CAD build for the part. Positions are in the model's coordinates, mm. Face numbers are marked on the shaded views. Round coordinates to 2 decimals unless told otherwise and drop trailing zeros. Order: outer loops, then holes, each group sorted by start corner. A loop starts at its lowest first (then second) coordinate and runs counter-clockwise, first axis right, second up. Notation, with made-up numbers: (21, -4.75) -> (67, -4.75) arc R22 ccw to (67, 32.25) -> close; hole circle Ø3 at (-39.5, 56). An arc over 180 degrees is marked (long way). Answer as CSV lines item,"result". Start each with the question number.
from build123d import *

# Parameters (mm, degrees)
SKETCH004_W          = 7
SKETCH004_H          = 3
SKETCH005_W          = 7
SKETCH005_H          = 3
POCKET_DEPTH         = 12.001
POCKET001_DEPTH      = 12.001
SKETCH009_W          = 7
SKETCH009_H          = 3
SKETCH010_W          = 7
SKETCH010_H          = 3
POCKET002_DEPTH      = 6.001
POCKET002_DEPTH_BACK = -6.001


with BuildPart() as part:
    # AdditivePipe: sweep along a path in Sketch002
    with BuildLine(Plane.XY) as additivepipe_path:
        ThreePointArc((0, 0), (-10.865453, 68.601773), (-42.398227, 130.488326))
    # Sketch → AdditivePipe (sweep)
    with BuildSketch(Plane.XZ):
        Polygon((-20, 6), (-20, -6), (-16, -6), (-16, -3), (-9, -3), (-9, -6), (9, -6), (9, -3), (16, -3), (16, -6), (20, -6), (20, 6), (16, 6), (16, 3), (9, 3), (9, 6), (-9, 6), (-9, 3), (-16, 3), (-16, 6), align=None)
    sweep(path=additivepipe_path.line)

    # AdditivePipe001: sweep along a path in Sketch001
    with BuildLine(Plane.XY) as additivepipe001_path:
        Line((0, 0), (0, 144))
    # Sketch → AdditivePipe001 (sweep)
    with BuildSketch(Plane.XZ):
        Polygon((-20, 6), (-20, -6), (-16, -6), (-16, -3), (-9, -3), (-9, -6), (9, -6), (9, -3), (16, -3), (16, -6), (20, -6), (20, 6), (16, 6), (16, 3), (9, 3), (9, 6), (-9, 6), (-9, 3), (-16, 3), (-16, 6), align=None)
    sweep(path=additivepipe001_path.line)

    # SubtractivePipe: sweep along a path in Sketch001
    with BuildLine(Plane.XY) as subtractivepipe_path:
        Line((0, 0), (0, 144))
    # Sketch004 → SubtractivePipe (sweep, cut)
    with BuildSketch(Plane.XZ):
        with Locations((-12.5, 4.5)):
            Rectangle(SKETCH004_W, SKETCH004_H)
    sweep(path=subtractivepipe_path.line, mode=Mode.SUBTRACT)

    # SubtractivePipe001: sweep along a path in Sketch002
    with BuildLine(Plane.XY) as subtractivepipe001_path:
        ThreePointArc((0, 0), (-10.865453, 68.601773), (-42.398227, 130.488326))
    # Sketch004 → SubtractivePipe001 (sweep, cut)
    with BuildSketch(Plane.XZ):
        with Locations((-12.5, 4.5)):
            Rectangle(SKETCH004_W, SKETCH004_H)
    sweep(path=subtractivepipe001_path.line, mode=Mode.SUBTRACT)

    # SubtractivePipe002: sweep along a path in Sketch002
    with BuildLine(Plane.XY) as subtractivepipe002_path:
        ThreePointArc((0, 0), (-10.865453, 68.601773), (-42.398227, 130.488326))
    # Sketch005 (on Face1 of SubtractivePipe001) → SubtractivePipe002 (sweep, cut)
    with BuildSketch(Plane.XZ):
        with Locations((12.5, 4.5)):
            Rectangle(SKETCH005_W, SKETCH005_H)
    sweep(path=subtractivepipe002_path.line, mode=Mode.SUBTRACT)

    # SubtractivePipe003: sweep along a path in Sketch001
    with BuildLine(Plane.XY) as subtractivepipe003_path:
        Line((0, 0), (0, 144))
    # Sketch005 (on Face1 of SubtractivePipe001) → SubtractivePipe003 (sweep, cut)
    with BuildSketch(Plane.XZ):
        with Locations((12.5, 4.5)):
            Rectangle(SKETCH005_W, SKETCH005_H)
    subtractivepipe003 = sweep(path=subtractivepipe003_path.line, mode=Mode.SUBTRACT)

    # Mirrored: SubtractivePipe003 across XY
    add(subtractivepipe003.mirror(Plane.XY), mode=Mode.SUBTRACT)

    # Sketch006 (on Face53 of Mirrored) → Pocket (cut, through all)
    with BuildSketch(Plane(origin=(0, 0, 6), x_dir=(-1, 0, 0), z_dir=(0, 0, 1))):
        with BuildLine():
            Line((38.757651, -133.13336), (46.038804, -127.843292))
            Line((46.038804, -127.843292), (41.924307, -122.180173))
            ThreePointArc((41.924307, -122.180173), (31.017586, -114.824218), (34.643154, -127.470241))
            Line((38.757651, -133.13336), (34.643154, -127.470241))
        make_face()
    extrude(amount=-POCKET_DEPTH, mode=Mode.SUBTRACT)

    # Sketch007 (on Face63 of Pocket) → Pocket001 (cut, through all)
    with BuildSketch(Plane(origin=(0, 0, 6), x_dir=(-1, 0, 0), z_dir=(0, 0, 1))):
        with BuildLine():
            Line((-4.5, -144), (4.5, -144))
            Line((4.5, -144), (4.5, -137))
            ThreePointArc((4.5, -137), (0, -124.638097), (-4.5, -137))
            Line((-4.5, -144), (-4.5, -137))
        make_face()
    extrude(amount=-POCKET001_DEPTH, mode=Mode.SUBTRACT)

    # SubtractivePipe004: sweep along a path in Sketch002
    with BuildLine(Plane.XY) as subtractivepipe004_path:
        ThreePointArc((0, 0), (-10.865453, 68.601773), (-42.398227, 130.488326))
    # Sketch009 → SubtractivePipe004 (sweep, cut)
    with BuildSketch(Plane.XZ):
        with Locations((-12.5, -4.5)):
            Rectangle(SKETCH009_W, SKETCH009_H)
    sweep(path=subtractivepipe004_path.line, mode=Mode.SUBTRACT)

    # SubtractivePipe005: sweep along a path in Sketch001
    with BuildLine(Plane.XY) as subtractivepipe005_path:
        Line((0, 0), (0, 144))
    # Sketch009 → SubtractivePipe005 (sweep, cut)
    with BuildSketch(Plane.XZ):
        with Locations((-12.5, -4.5)):
            Rectangle(SKETCH009_W, SKETCH009_H)
    sweep(path=subtractivepipe005_path.line, mode=Mode.SUBTRACT)

    # SubtractivePipe006: sweep along a path in Sketch002
    with BuildLine(Plane.XY) as subtractivepipe006_path:
        ThreePointArc((0, 0), (-10.865453, 68.601773), (-42.398227, 130.488326))
    # Sketch010 (on Face1 of SubtractivePipe005) → SubtractivePipe006 (sweep, cut)
    with BuildSketch(Plane.XZ):
        with Locations((12.5, -4.5)):
            Rectangle(SKETCH010_W, SKETCH010_H)
    sweep(path=subtractivepipe006_path.line, mode=Mode.SUBTRACT)

    # Sketch011 → Pocket002 (cut, two sides)
    with BuildSketch(Plane.XY) as pocket002_sk:
        with BuildLine():
            Line((-4.5, 0), (4.5, 0))
            Line((4.5, 0), (4.5, 7))
            ThreePointArc((4.5, 7), (0, 19.361903), (-4.5, 7))
            Line((-4.5, 0), (-4.5, 7))
        make_face()
    extrude(amount=-POCKET002_DEPTH, mode=Mode.SUBTRACT)
    extrude(pocket002_sk.sketch, amount=-POCKET002_DEPTH_BACK, mode=Mode.SUBTRACT)


solid = part.part
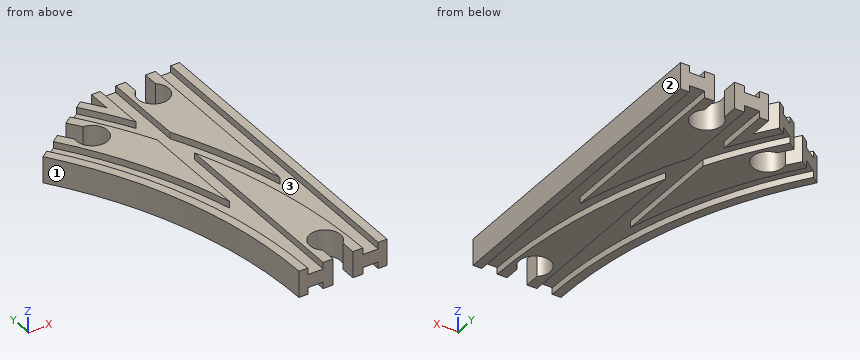
Item 1: Band-saw the part on B-B, the plane x = 14. Give the cut face in (y, z), and give its area (3 significant figures).
Item 2: Probe line 1 (X direction, y = 101.5, z = -4.25); line 2 (X direction, y = 107, z = 3.25); line 3 (X direction, y = 36, z = -3.75). List the from-to ranges inside material, lowest first.
Item 3: Band-saw the part on A-A, the plane z = 4.5. Count the separate pieces of the cut face and the enclosed holes in it, and give its area (3 significant figures).
Item 4: Mould opens along Y. For the marked faces 1, 2 and 3 say: released by +Y, released by -Y, zero draft, split by the parting line, or undercut.
Item 5: Band-saw the part on C-C, the plane y = 31. Give the cut face in (x, z), and give its area (3 significant figures).
Item 6: Pin check, flat tips, straight feed: pin 1 (2.5 mm diameter, centred on y = 28, z = -4, fed in from -X); pin 2 (1.5 mm diameter, centred on y = 57.5, z = 4, fed in from -X); pin 3 (2 mm diameter, centred on y = 140, z = 2, fed in from -X). Stop position of each tip, or through.
Item 7: Band-saw the part on D-D, the plane x = 0. Give the cut face in (y, z).
Values:
1,outline,"(0, -3) -> (144, -3) -> (144, 3) -> (0, 3) -> close"
1,area,"864 mm²"
2,line 1,"-47.35 to -42.74, -34.74 to -16, -6.73 to 9, 16 to 20"
2,line 2,"-50.67 to -45.97, -37.83 to -17.28, -9 to 9, 16 to 20"
2,line 3,"-23.23 to -19.17, -9 to 6.18, 16 to 20"
3,separate pieces,"6"
3,enclosed holes,"0"
3,area,"3,760 mm²"
4,face 1,"released by -Y"
4,face 2,"zero draft"
4,face 3,"undercut"
5,outline,"(-22.39, -6) -> (-18.35, -6) -> (-18.35, -3) -> (-9, -3) -> (-9, -6) -> (6.91, -6) -> (6.91, -3) -> (16, -3) -> (16, -6) -> (20, -6) -> (20, 6) -> (16, 6) -> (16, 3) -> (6.91, 3) -> (6.91, 6) -> (-9, 6) -> (-9, 3) -> (-18.35, 3) -> (-18.35, 6) -> (-22.39, 6) -> close"
5,area,"398 mm²"
6,pin 1,"x = -22.13"
6,pin 2,"x = -28.58"
6,pin 3,"x = -30.68"
7,outline,"(19.36, -6) -> (63.85, -6) -> (63.85, -3) -> (85.79, -3) -> (85.79, -6) -> (124.64, -6) -> (124.64, 6) -> (85.79, 6) -> (85.79, 3) -> (63.85, 3) -> (63.85, 6) -> (19.36, 6) -> close"
